Can you work these out from the model? Positions are in its coordinate system, mm. Give positions to 0.01 mm unless a question says otherwise; leave off trailing zeros. Write each loop counter-clockwise with the first axis right and the second up, starting at its lowest first coordinate (ties: lowest second). Pieces come first, ordered by that corner, then holes.
```python
from build123d import *

# Parameters (mm, degrees)
COMPUTE_COMBO_PLATE_W   = 160
COMPUTE_COMBO_PLATE_H   = 170
COMPUTE_COMBO_PLATE_R   = 1.45
COMPUTE_COMBO_PLATE_W_2 = 48
COMPUTE_COMBO_PLATE_H_2 = 34
F_3MM_DEPTH             = 3


with BuildPart() as part:
    # 外形与孔位_compute_combo_plate → 板厚_3mm (new body)
    with BuildSketch(Plane.XY):
        with Locations((80, 85)):
            Rectangle(COMPUTE_COMBO_PLATE_W, COMPUTE_COMBO_PLATE_H)
        with Locations((51, 80.5)):
            Circle(COMPUTE_COMBO_PLATE_R, mode=Mode.SUBTRACT)
        with Locations((51, 129.5)):
            Circle(COMPUTE_COMBO_PLATE_R, mode=Mode.SUBTRACT)
        with Locations((109, 80.5)):
            Circle(COMPUTE_COMBO_PLATE_R, mode=Mode.SUBTRACT)
        with Locations((109, 129.5)):
            Circle(COMPUTE_COMBO_PLATE_R, mode=Mode.SUBTRACT)
        with Locations((37, 76)):
            Circle(COMPUTE_COMBO_PLATE_R, mode=Mode.SUBTRACT)
        with Locations((37, 134)):
            Circle(COMPUTE_COMBO_PLATE_R, mode=Mode.SUBTRACT)
        with Locations((123, 76)):
            Circle(COMPUTE_COMBO_PLATE_R, mode=Mode.SUBTRACT)
        with Locations((123, 134)):
            Circle(COMPUTE_COMBO_PLATE_R, mode=Mode.SUBTRACT)
        with Locations((80, 105)):
            Rectangle(COMPUTE_COMBO_PLATE_W_2, COMPUTE_COMBO_PLATE_H_2, mode=Mode.SUBTRACT)
        with BuildLine():
            Line((19.75, 22.75), (40.25, 22.75))
            ThreePointArc((40.25, 22.75), (43, 20), (40.25, 17.25))
            Line((40.25, 17.25), (19.75, 17.25))
            ThreePointArc((19.75, 17.25), (17, 20), (19.75, 22.75))
        make_face(mode=Mode.SUBTRACT)
        with BuildLine():
            Line((119.75, 22.75), (140.25, 22.75))
            ThreePointArc((140.25, 22.75), (143, 20), (140.25, 17.25))
            Line((140.25, 17.25), (119.75, 17.25))
            ThreePointArc((119.75, 17.25), (117, 20), (119.75, 22.75))
        make_face(mode=Mode.SUBTRACT)
    extrude(amount=F_3MM_DEPTH)


solid = part.part
```
1) Please list where these lines run through material, in increasing order: L1, parallel to Y at x = 51, z = 1.15; L2, parallel to X at y = 134, z = 1.25; L3, parallel to X at y = 129.5, z = 2.25.
Values follow:
L1: y = 0 to 79.05, 81.95 to 128.05, 130.95 to 170
L2: x = 0 to 35.55, 38.45 to 121.55, 124.45 to 160
L3: x = 0 to 49.55, 52.45 to 107.55, 110.45 to 160
2) For pin 1 Ø1.7 at (x, y) = (51, 129.5) entering from -Z, with a flat end and sliding along its axis, tell me the tip position at first contact or that it passes through.
Values follow:
pin 1: passes through
3) Suppose I cut it at A-A on y = 115. Write out the boundary of the cut face in (x, z), plus the area to 3 significant figures.
Values follow:
outline: (0, 0) - (56, 0) - (56, 3) - (0, 3) - close; (104, 0) - (160, 0) - (160, 3) - (104, 3) - close
area: 336 mm2
4) Suppose I cut it at B-B on x = 138. Write out the boundary of the cut face in (y, z), plus the area to 4 significant figures.
Values follow:
outline: (0, 0) - (17.25, 0) - (17.25, 3) - (0, 3) - close; (22.75, 0) - (170, 0) - (170, 3) - (22.75, 3) - close
area: 493.5 mm2
5) Suppose I cut it at D-D on z = 1.35. State how many separate pieces and enclosed holes the cut face has, plus the area to 3 significant figures.
Values follow:
separate pieces: 1
enclosed holes: 11
area: 25,200 mm2
6) Suppose I cut it at C-C on y = 20. Write out the boundary of the cut face in (x, z), plus the area to 3 significant figures.
Values follow:
outline: (0, 0) - (17, 0) - (17, 3) - (0, 3) - close; (43, 0) - (117, 0) - (117, 3) - (43, 3) - close; (143, 0) - (160, 0) - (160, 3) - (143, 3) - close
area: 324 mm2
